```python
from build123d import *

# Parameters (mm, degrees)
F0_R     = 1.1
F0_R_2   = 3
F1_DEPTH = 1


with BuildPart() as f1:
    # F0 (on Front) → F1 (new body)
    with BuildSketch(Plane.XZ):
        with BuildLine():
            ThreePointArc((-5.59017, -3), (-4.773673, -3.174258), (-4.099458, -3.666667))
            ThreePointArc((-4.099458, -3.666667), (5.5, 0), (-4.099458, 3.666667))
            ThreePointArc((-4.099458, 3.666667), (-4.773673, 3.174258), (-5.59017, 3))
            Line((-5.59017, 3), (-50, 3))
            ThreePointArc((-50, 3), (-53, 0), (-50, -3))
            Line((-50, -3), (-5.59017, -3))
        make_face()
        with Locations((-50, 0)):
            Circle(F0_R, mode=Mode.SUBTRACT)
        with Locations((-23, 0)):
            Circle(F0_R, mode=Mode.SUBTRACT)
        Circle(F0_R_2, mode=Mode.SUBTRACT)
    extrude(amount=F1_DEPTH)


solid = f1.part
```
Source: CAD feature listing. Evaluate the final solid. Frame: model axes, mm. A direction names the side the tool comes from. Give positions to 0.01 mm unless a question says otherwise; leave off trailing zeros. Loops run counter-clockwise (first coordinate to the right, second up) from the corner with the lowest first, then second, coordinate; pieces in that order, holes last. Notation, with made-up numbers: (7, -19.5) - (33, -19.5) arc R35 cw to (33, 13.5) - close; hole circle Ø5 at (64, -29.75). An arc over 180 degrees is marked (long way). Use CSV: the item, a comma, the result in double quotes. Start each with the question number.
1. Section A-A (x = -23). Output: boundary loops of the cut face in (y, z), then the cut area to 3 significant figures.
2. Section B-B (z = 0). Output: boundary loops of the cut face in (x, y).
3. Draft query along Z for faces 1 (the flat face through (-24, 0, 1)), 2 (the cylindrical face through (-53, -0.5, 0.1)), 3 (the cylindrical face through (-24.1, -0.5, 0)). Return one class per face: +Z half, -Z half, draft (parallel to the pull), parting line (faces both ways), or undercut.
4. Pin query (flat end, axial travel): pin 1 (0.5 mm diameter, centred on x = -27, y = -0.5, fed in from -Z). Return the tip coordinate at first contact, or that it passes through.
5. Section C-C (y = -0.5). Output: boundary loops of the cut face in (x, z).
6. Ray query, L1, parallel to Z at x = 0, y = -0.2; L2, parallel to Z at x = -23, y = -0.4; L3, parallel to Z at x = -41, y = -0.45. Return the intervals inside material, ascending.
7. Reachability of faces 4 (the flat face through (-28.1, -0.5, -3)), 5 (the cylindrical face through (-51.1, -0.5, 0)), 6 (the flat face through (-27.5, -0.5, 3)) from +Z, -Z, +X, -X, +Y, -Y: full face, straight path, thin tool, end or side. Return the list, or none.
8. Section D-D (x = 0). Output: boundary loops of the cut face in (y, z), then the cut area to 3 significant figures.
Response:
1,outline,"(-1, -3) - (0, -3) - (0, -1.1) - (-1, -1.1) - close; (-1, 1.1) - (0, 1.1) - (0, 3) - (-1, 3) - close"
1,area,"3.80 mm²"
2,outline,"(-53, -1) - (-51.1, -1) - (-51.1, 0) - (-53, 0) - close; (-48.9, -1) - (-24.1, -1) - (-24.1, 0) - (-48.9, 0) - close; (-21.9, -1) - (-3, -1) - (-3, 0) - (-21.9, 0) - close; (3, -1) - (5.5, -1) - (5.5, 0) - (3, 0) - close"
3,face 1,"draft"
3,face 2,"parting line"
3,face 3,"undercut"
4,pin 1,"z = -3"
5,outline,"(-50, -3) - (-5.59, -3) arc R2 cw to (-4.1, -3.67) arc R5.5 ccw (long way) to (-4.1, 3.67) arc R2 cw to (-5.59, 3) - (-50, 3) arc R3 ccw to start; hole circle Ø2.2 at (-50, 0); hole circle Ø2.2 at (-23, 0); hole circle Ø6 at (0, 0)"
6,L1,"-5.5 to -3, 3 to 5.5"
6,L2,"-3 to -1.1, 1.1 to 3"
6,L3,"-3 to 3"
7,face 4,"-Z, -X, +Y, -Y"
7,face 5,"+Y, -Y"
7,face 6,"+Z, -X, +Y, -Y"
8,outline,"(-1, -5.5) - (0, -5.5) - (0, -3) - (-1, -3) - close; (-1, 3) - (0, 3) - (0, 5.5) - (-1, 5.5) - close"
8,area,"5.00 mm²"
